Design review of the part built by this model. Coordinates are the model's own, in mm. Face numbers are marked on the shaded views. A direction names the side the tool comes from. Round coordinates to 2 decimals unless told otherwise and drop trailing zeros. Write each loop counter-clockwise with the first axis right and the second up, starting at its lowest first coordinate (ties: lowest second). Pieces come first, ordered by that corner, then holes. Notation, with made-up numbers: (70, 5.5) - (120, 5.5) arc R21 ccw to (120, 14.5) - close; hole circle Ø2 at (51.5, 31). An arc over 180 degrees is marked (long way). Use one line per item in the form item = value.
```python
from build123d import *

# Parameters (mm, degrees)
BOSS_EXTRUDE1_DEPTH = 2
BOSS_EXTRUDE2_DEPTH = 31
CUT_EXTRUDE1_DEPTH  = 56.481979056
CUT_EXTRUDE2_DEPTH  = 56.481979228
SKETCH5_R           = 3.2
CUT_EXTRUDE3_DEPTH  = 56.481979228
SKETCH6_R           = 5
CUT_EXTRUDE4_DEPTH  = 56.481979228


with BuildPart() as part:
    # Sketch1 → Boss-Extrude1 (new body)
    with BuildSketch(Plane.XY):
        with BuildLine():
            Line((0, 0), (0, 22))
            ThreePointArc((0, 22), (13.5, 35.5), (27, 22))
            Line((27, 22), (27, 0))
            Line((27, 0), (0, 0))
        make_face()
    extrude(amount=BOSS_EXTRUDE1_DEPTH)

    # Sketch2 → Boss-Extrude2 (add)
    with BuildSketch(Plane.XY.offset(2)):
        with BuildLine():
            Line((27, 0), (27, 22))
            ThreePointArc((27, 22), (13.5, 35.5), (0, 22))
            Line((0, 22), (0, 0))
            Line((0, 0), (1.5, 0))
            Line((1.5, 0), (1.5, 1.5))
            Line((1.5, 1.5), (1.5, 22))
            ThreePointArc((1.5, 22), (13.5, 34), (25.5, 22))
            Line((25.5, 22), (25.5, 1.5))
            Line((25.5, 1.5), (25.5, 0))
            Line((25.5, 0), (27, 0))
        make_face()
    extrude(amount=BOSS_EXTRUDE2_DEPTH)

    # Sketch3 → Cut-Extrude1 (cut, through all)
    with BuildSketch(Plane(origin=(0, 0, 0), x_dir=(1, 0, 0), z_dir=(0, 1, 0))):
        with BuildLine():
            Line((1.5, -33), (1.5, -16))
            ThreePointArc((1.5, -16), (13.5, -4), (25.5, -16))
            Line((25.5, -16), (25.5, -33))
            Line((25.5, -33), (1.5, -33))
        make_face()
    extrude(amount=CUT_EXTRUDE1_DEPTH, mode=Mode.SUBTRACT)

    # Sketch4 → Cut-Extrude2 (cut, through all)
    with BuildSketch(Plane.ZY):
        with BuildLine():
            Line((33, 31.363603565), (9.117273512, 31.363603565))
            add(Edge.make_bspline(
                [(9.117273512, 31.363603565), (12.96325336, 25.746828887), (19.327266499, 25.020144715), (24.670979231, 22)],
                knots=[0, 0, 0, 0, 0.522970266, 0.522970266, 0.522970266, 0.522970266], degree=3))
            Line((24.670979231, 22), (33, 22))
            Line((33, 22), (33, 31.363603565))
        make_face()
        with BuildLine():
            Line((33, 22), (24.670979231, 22))
            add(Edge.make_bspline(
                [(24.670979231, 22), (28.91814661, 19.599597741), (32.520787743, 15.750410887), (33, 10.690145811)],
                knots=[0.522970266, 0.522970266, 0.522970266, 0.522970266, 0.938625516, 0.938625516, 0.938625516, 0.938625516], degree=3))
            Line((33, 10.690145811), (33, 22))
        make_face()
    extrude(amount=-CUT_EXTRUDE2_DEPTH, mode=Mode.SUBTRACT)

    # Sketch5 → Cut-Extrude3 (cut, through all)
    with BuildSketch(Plane.ZY):
        with Locations((26.5, 5)):
            Circle(SKETCH5_R)
    extrude(amount=-CUT_EXTRUDE3_DEPTH, mode=Mode.SUBTRACT)

    # Sketch6 → Cut-Extrude4 (cut, through all)
    with BuildSketch(Plane(origin=(0, 0, 0), x_dir=(-1, 0, 0), z_dir=(0, 0, -1))):
        with Locations((-13.5, 23.5)):
            Circle(SKETCH6_R)
    extrude(amount=-CUT_EXTRUDE4_DEPTH, mode=Mode.SUBTRACT)


solid = part.part
```
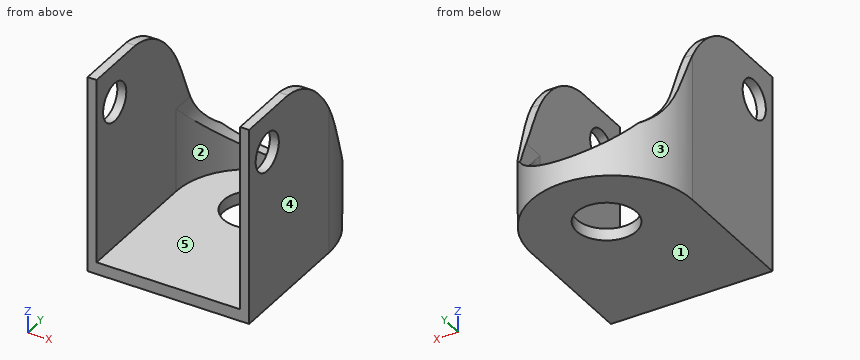
Q1. We need section A-A on y = 5. Write out the cut boundary in (x, z), then the cut area to 3 significant figures.
Calculated:
outline = (0, 0) - (27, 0) - (27, 23.3) - (25.5, 23.3) - (25.5, 2) - (1.5, 2) - (1.5, 23.3) - (0, 23.3) - close; (0, 29.7) - (1.5, 29.7) - (1.5, 33) - (0, 33) - close; (25.5, 29.7) - (27, 29.7) - (27, 33) - (25.5, 33) - close
area = 128 mm2
Q2. We need section D-D on x = 13.5. Write out the cut boundary in (y, z), then the cut area to 3 significant figures.
Calculated:
outline = (0, 0) - (18.5, 0) - (18.5, 2) - (0, 2) - close; (28.5, 0) - (35.5, 0) - (35.5, 4) - (34, 4) - (34, 2) - (28.5, 2) - close
area = 54.0 mm2
Q3. Machinability: for the marked faces 4 and 5, which of the approach directions +Z, -Z, +X, -X, +Y, -Y give a long, thin tool a straight path to every point of the face, cutting with its end or side? Answer none if there is none.
Calculated:
face_4 = +Z, -Z, +X, +Y, -Y
face_5 = +Z, -Y
Q4. For P1, Ø12, axis at x = 9, y = 30.5, coming from the +Z side; P2, Ø12, axis at x = 8, y = 10.5, coming from the +Z side, all flat-tipped, find the tip position at first contact; note any pin that passes through.
Calculated:
P1 = 10.16
P2 = 2
Q5. We need section C-C on z = 2.5. Write out the cut boundary in (x, y), then the cut area to 3 significant figures.
Calculated:
outline = (0, 0) - (1.5, 0) - (1.5, 22) arc R12 cw to (25.5, 22) - (25.5, 0) - (27, 0) - (27, 22) arc R13.5 ccw to (0, 22) - close
area = 126 mm2
Q6. We need section B-B on x = 10.25. Write out the cut boundary in (y, z), then the cut area to 3 significant figures.
Calculated:
outline = (0, 0) - (19.7, 0) - (19.7, 2) - (0, 2) - close; (27.3, 0) - (35.1, 0) - (35.1, 4.45) - (33.55, 4.45) - (33.55, 2) - (27.3, 2) - close
area = 58.8 mm2
Q7. To check wall thickness, follow line 1 along X through (y, z) = (9, 6.5); line 2 along Y through (x, z) = (13.5, 1.4); line 3 along Z through (x, y) = (10.5, 10.5). State the ranges of each line that lie inside material, in increasing order. Write a range as from..to.
Calculated:
line_1 = 0..1.5, 25.5..27
line_2 = 0..18.5, 28.5..35.5
line_3 = 0..2
Q8. Draft analysis for pull direction X (two halves, no side actions). For the marked faces 1, 2 and 3, state which applies: released by +X, released by -X, zero draft, split by the parting line, or undercut.
Calculated:
face_1 = zero draft
face_2 = undercut
face_3 = split by the parting line
